Could you check a few things on this model? Use its own coordinates, in mm. Coordinates: 2 decimals unless noted, no trailing zeros. Loops run counter-clockwise (first coordinate to the right, second up) from the corner with the lowest first, then second, coordinate; pieces in that order, holes last. Notation, with made-up numbers: (-4, 45.5) - (5, 45.5) arc R15 ccw to (5, 52.5) - close; hole circle Ø11 at (-29, -32.5). An arc over 180 degrees is marked (long way). One line per item, written item: value. Start each with the question number.
(1) If we mould it in two halves opening along X, with no side actions, what happens to faces 1 (the face through (-6.94, -30.24, -42.03)), 2 (the face through (26.92, -11.594, -42.028)), 3 (the face through (10.59, -24.38, -42.03)), 4 (the face through (-0.1, 27.2, -44))? For each: pulls with the +X half, pulls with the -X half, needs draft (parallel to the pull), parting line crosses it, or undercut.
(2) If we section it at D-D on x = -26.79: Write out the boundary of the cut face in (y, z), then the cut area to 3 significant figures.
(3) If I drill on line 1 along Y through (x, z) = (-11.1, -41.6); line 2 along Y through (x, z) = (-27.5, -43); line 3 along X through (y, z) = (12.1, -41.35), over which ranges is the centre line in solid material (lowest first)? Write a range as from..to.
(4) If we section it at C-C on z = -42.2: Count the separate pieces of the cut face and the enclosed holes in it, then the cut area to 3 significant figures.
(5) I'm going to push flat-ended pins straight in: P1, Ø1, axis at x = 17.5, z = -41, coming from the -Y side; P2, Ø1, axis at y = -20.5, z = -40.5, coming from the +X side. Where does each tip first touch, or does it pass through?
(6) If we section it at A-A on y = 1: Write out the boundary of the cut face in (x, z).
(7) If we section it at B-B on x = 0: Write out the boundary of the cut face in (y, z), then the cut area to 3 significant figures.
```python
from build123d import *

# Parameters (mm, degrees)
CYLINDER1907_R               = 3
CYLINDER1907_DEPTH           = 3
CYLINDER1907_PLACEMENT_ANGLE = 67.5
CYLINDER1905_R               = 3
CYLINDER1905_DEPTH           = 3
CYLINDER1905_PLACEMENT_ANGLE = 112.5
CYLINDER1297_R               = 3
CYLINDER1297_DEPTH           = 3
CYLINDER1297_PLACEMENT_ANGLE = 157.5
CYLINDER1908_R               = 3
CYLINDER1908_DEPTH           = 3
CYLINDER1908_PLACEMENT_ANGLE = 202.5
CYLINDER1296_R               = 3
CYLINDER1296_DEPTH           = 3
CYLINDER1296_PLACEMENT_ANGLE = 112.5
CYLINDER1906_R               = 3
CYLINDER1906_DEPTH           = 3
CYLINDER1906_PLACEMENT_ANGLE = 67.5
CYLINDER1298_R               = 3
CYLINDER1298_DEPTH           = 3
CYLINDER1298_PLACEMENT_ANGLE = 22.5
CYLINDER1904_R               = 3
CYLINDER1904_DEPTH           = 3
CYLINDER1904_PLACEMENT_ANGLE = 22.5
CYLINDER1896_R               = 1.5
CYLINDER1896_DEPTH           = 20
CYLINDER1896_PLACEMENT_ANGLE = 67.5
CYLINDER1899_R               = 1.5
CYLINDER1899_DEPTH           = 20
CYLINDER1899_PLACEMENT_ANGLE = 112.5
CYLINDER1902_R               = 1.5
CYLINDER1902_DEPTH           = 20
CYLINDER1902_PLACEMENT_ANGLE = 157.5
CYLINDER1903_R               = 1.5
CYLINDER1903_DEPTH           = 20
CYLINDER1903_PLACEMENT_ANGLE = 202.5
CYLINDER1900_R               = 1.5
CYLINDER1900_DEPTH           = 20
CYLINDER1900_PLACEMENT_ANGLE = 112.5
CYLINDER1897_R               = 1.5
CYLINDER1897_DEPTH           = 20
CYLINDER1897_PLACEMENT_ANGLE = 67.5
CYLINDER1901_R               = 1.5
CYLINDER1901_DEPTH           = 20
CYLINDER1901_PLACEMENT_ANGLE = 22.5
CYLINDER1898_R               = 1.5
CYLINDER1898_DEPTH           = 20
CYLINDER1898_PLACEMENT_ANGLE = 22.5
TUBE012_R                    = 32
TUBE012_R_2                  = 26
TUBE012_DEPTH                = 4


with BuildPart() as obj1:
    # Cylinder1907 → Cylinder1907 (new body)
    with BuildSketch(Plane.XY):
        Circle(CYLINDER1907_R)
    extrude(amount=CYLINDER1907_DEPTH)


with BuildPart() as obj1_1:
    # Cylinder1907 placement: moved
    add(obj1.part.moved(Location((11.1, 26.79, -50))).rotate(Axis((11.1, 26.79, -50), (0, 0, 1)), CYLINDER1907_PLACEMENT_ANGLE))


with BuildPart() as obj2:
    # Cylinder1905 → Cylinder1905 (new body)
    with BuildSketch(Plane.XY):
        Circle(CYLINDER1905_R)
    extrude(amount=CYLINDER1905_DEPTH)


with BuildPart() as obj2_1:
    # Cylinder1905 placement: moved
    add(obj2.part.moved(Location((-11.1, 26.79, -50))).rotate(Axis((-11.1, 26.79, -50), (0, 0, 1)), CYLINDER1905_PLACEMENT_ANGLE))


with BuildPart() as obj3:
    # Cylinder1297 → Cylinder1297 (new body)
    with BuildSketch(Plane.XY):
        Circle(CYLINDER1297_R)
    extrude(amount=CYLINDER1297_DEPTH)


with BuildPart() as obj3_1:
    # Cylinder1297 placement: moved
    add(obj3.part.moved(Location((-26.79, 11.1, -50))).rotate(Axis((-26.79, 11.1, -50), (0, 0, 1)), CYLINDER1297_PLACEMENT_ANGLE))


with BuildPart() as obj4:
    # Cylinder1908 → Cylinder1908 (new body)
    with BuildSketch(Plane.XY):
        Circle(CYLINDER1908_R)
    extrude(amount=CYLINDER1908_DEPTH)


with BuildPart() as obj4_1:
    # Cylinder1908 placement: moved
    add(obj4.part.moved(Location((-26.79, -11.1, -50))).rotate(Axis((-26.79, -11.1, -50), (0, 0, 1)), CYLINDER1908_PLACEMENT_ANGLE))


with BuildPart() as obj5:
    # Cylinder1296 → Cylinder1296 (new body)
    with BuildSketch(Plane.XY):
        Circle(CYLINDER1296_R)
    extrude(amount=CYLINDER1296_DEPTH)


with BuildPart() as obj5_1:
    # Cylinder1296 placement: moved
    add(obj5.part.moved(Location((-11.1, -26.79, -50))).rotate(Axis((-11.1, -26.79, -50), (0, 0, -1)), CYLINDER1296_PLACEMENT_ANGLE))


with BuildPart() as obj6:
    # Cylinder1906 → Cylinder1906 (new body)
    with BuildSketch(Plane.XY):
        Circle(CYLINDER1906_R)
    extrude(amount=CYLINDER1906_DEPTH)


with BuildPart() as obj6_1:
    # Cylinder1906 placement: moved
    add(obj6.part.moved(Location((11.1, -26.79, -50))).rotate(Axis((11.1, -26.79, -50), (0, 0, -1)), CYLINDER1906_PLACEMENT_ANGLE))


with BuildPart() as obj7:
    # Cylinder1298 → Cylinder1298 (new body)
    with BuildSketch(Plane.XY):
        Circle(CYLINDER1298_R)
    extrude(amount=CYLINDER1298_DEPTH)


with BuildPart() as obj7_1:
    # Cylinder1298 placement: moved
    add(obj7.part.moved(Location((26.79, -11.1, -50))).rotate(Axis((26.79, -11.1, -50), (0, 0, -1)), CYLINDER1298_PLACEMENT_ANGLE))


with BuildPart() as compound856:
    # Cylinder1904 → Cylinder1904 (new body)
    with BuildSketch(Plane.XY):
        Circle(CYLINDER1904_R)
    extrude(amount=CYLINDER1904_DEPTH)


with BuildPart() as compound856_1:
    # Cylinder1904 placement: moved
    add(compound856.part.moved(Location((26.79, 11.1, -50))).rotate(Axis((26.79, 11.1, -50), (0, 0, 1)), CYLINDER1904_PLACEMENT_ANGLE))

    # Compound856: union obj1, obj2, obj3, obj4, obj5, obj6, obj7
    add(obj1_1.part)
    add(obj2_1.part)
    add(obj3_1.part)
    add(obj4_1.part)
    add(obj5_1.part)
    add(obj6_1.part)
    add(obj7_1.part)


with BuildPart() as obj8:
    # Cylinder1896 → Cylinder1896 (new body)
    with BuildSketch(Plane.XY):
        Circle(CYLINDER1896_R)
    extrude(amount=CYLINDER1896_DEPTH)


with BuildPart() as obj8_1:
    # Cylinder1896 placement: moved
    add(obj8.part.moved(Location((11.1, 26.79, -50))).rotate(Axis((11.1, 26.79, -50), (0, 0, 1)), CYLINDER1896_PLACEMENT_ANGLE))


with BuildPart() as obj9:
    # Cylinder1899 → Cylinder1899 (new body)
    with BuildSketch(Plane.XY):
        Circle(CYLINDER1899_R)
    extrude(amount=CYLINDER1899_DEPTH)


with BuildPart() as obj9_1:
    # Cylinder1899 placement: moved
    add(obj9.part.moved(Location((-11.1, 26.79, -50))).rotate(Axis((-11.1, 26.79, -50), (0, 0, 1)), CYLINDER1899_PLACEMENT_ANGLE))


with BuildPart() as obj10:
    # Cylinder1902 → Cylinder1902 (new body)
    with BuildSketch(Plane.XY):
        Circle(CYLINDER1902_R)
    extrude(amount=CYLINDER1902_DEPTH)


with BuildPart() as obj10_1:
    # Cylinder1902 placement: moved
    add(obj10.part.moved(Location((-26.79, 11.1, -50))).rotate(Axis((-26.79, 11.1, -50), (0, 0, 1)), CYLINDER1902_PLACEMENT_ANGLE))


with BuildPart() as obj11:
    # Cylinder1903 → Cylinder1903 (new body)
    with BuildSketch(Plane.XY):
        Circle(CYLINDER1903_R)
    extrude(amount=CYLINDER1903_DEPTH)


with BuildPart() as obj11_1:
    # Cylinder1903 placement: moved
    add(obj11.part.moved(Location((-26.79, -11.1, -50))).rotate(Axis((-26.79, -11.1, -50), (0, 0, 1)), CYLINDER1903_PLACEMENT_ANGLE))


with BuildPart() as obj12:
    # Cylinder1900 → Cylinder1900 (new body)
    with BuildSketch(Plane.XY):
        Circle(CYLINDER1900_R)
    extrude(amount=CYLINDER1900_DEPTH)


with BuildPart() as obj12_1:
    # Cylinder1900 placement: moved
    add(obj12.part.moved(Location((-11.1, -26.79, -50))).rotate(Axis((-11.1, -26.79, -50), (0, 0, -1)), CYLINDER1900_PLACEMENT_ANGLE))


with BuildPart() as obj13:
    # Cylinder1897 → Cylinder1897 (new body)
    with BuildSketch(Plane.XY):
        Circle(CYLINDER1897_R)
    extrude(amount=CYLINDER1897_DEPTH)


with BuildPart() as obj13_1:
    # Cylinder1897 placement: moved
    add(obj13.part.moved(Location((11.1, -26.79, -50))).rotate(Axis((11.1, -26.79, -50), (0, 0, -1)), CYLINDER1897_PLACEMENT_ANGLE))


with BuildPart() as obj14:
    # Cylinder1901 → Cylinder1901 (new body)
    with BuildSketch(Plane.XY):
        Circle(CYLINDER1901_R)
    extrude(amount=CYLINDER1901_DEPTH)


with BuildPart() as obj14_1:
    # Cylinder1901 placement: moved
    add(obj14.part.moved(Location((26.79, -11.1, -50))).rotate(Axis((26.79, -11.1, -50), (0, 0, -1)), CYLINDER1901_PLACEMENT_ANGLE))


with BuildPart() as compound855:
    # Cylinder1898 → Cylinder1898 (new body)
    with BuildSketch(Plane.XY):
        Circle(CYLINDER1898_R)
    extrude(amount=CYLINDER1898_DEPTH)


with BuildPart() as compound855_1:
    # Cylinder1898 placement: moved
    add(compound855.part.moved(Location((26.79, 11.1, -50))).rotate(Axis((26.79, 11.1, -50), (0, 0, 1)), CYLINDER1898_PLACEMENT_ANGLE))

    # Compound855: union obj8, obj9, obj10, obj11, obj12, obj13, obj14
    add(obj8_1.part)
    add(obj9_1.part)
    add(obj10_1.part)
    add(obj11_1.part)
    add(obj12_1.part)
    add(obj13_1.part)
    add(obj14_1.part)


with BuildPart() as t_mini_washer:
    # Tube012 → Tube012 (new body)
    with BuildSketch(Plane.XY.offset(-47)):
        Circle(TUBE012_R)
        Circle(TUBE012_R_2, mode=Mode.SUBTRACT)
    extrude(amount=TUBE012_DEPTH)

    # Cut692: cut Compound855
    add(compound855_1.part, mode=Mode.SUBTRACT)


with BuildPart() as t_mini_washer_1:
    # Cut692 placement: moved
    add(t_mini_washer.part.moved(Location((0, 0, 2))))

    # Cut693: cut Compound856
    add(compound856_1.part, mode=Mode.SUBTRACT)


with BuildPart() as t_mini_washer_2:
    # Cut693 placement: moved
    add(t_mini_washer_1.part.moved(Location((0, 1, 1))))


solid = t_mini_washer_2.part
```
Values:
1. face 1: parting line crosses it
1. face 2: undercut
1. face 3: undercut
1. face 4: needs draft
2. outline: (-16.5, -44) - (-11.6, -44) - (-11.6, -40) - (-16.5, -40) - close; (-8.6, -44) - (10.6, -44) - (10.6, -40) - (-8.6, -40) - close; (13.6, -44) - (18.5, -44) - (18.5, -40) - (13.6, -40) - close
2. area: 116 mm2
3. line 1: y = -29.01..-27.29, -24.29..-22.51, 24.51..26.29, 29.29..31.01
3. line 2: y = -15.36..-11.42, -8.78..10.78, 13.42..17.36
3. line 3: x = -30.01..-28.29, -25.29..-23.51, 23.51..25.29, 28.29..30.01
4. separate pieces: 1
4. enclosed holes: 9
4. area: 1,040 mm2
5. P1: stops at y = -26.11
5. P2: stops at x = 24.15
6. outline: (-32, -44) - (-26, -44) - (-26, -40) - (-32, -40) - close; (26, -44) - (32, -44) - (32, -40) - (26, -40) - close
7. outline: (-31, -44) - (-25, -44) - (-25, -40) - (-31, -40) - close; (27, -44) - (33, -44) - (33, -40) - (27, -40) - close
7. area: 48.0 mm2
